```python
from build123d import *

# Parameters (mm, degrees)
F1_DEPTH = 25


with BuildPart() as f1:
    # F0 (on Right) → F1 (new body, symmetric)
    with BuildSketch(Plane.YZ):
        Polygon((-25, 0), (25, 0), (25, 45), (44.870459, 45), (44.870459, 60), (25, 60), (17, 103.547319), (25, 103.547319), (25, 121.547319), (-5, 121.547319), (-25, 91.547319), align=None)
    extrude(amount=F1_DEPTH, both=True)


solid = f1.part
```
Geometry: final body of the model. Coordinates: model frame, mm. A direction names the side the tool comes from. Coordinates: 2 decimals unless noted, no trailing zeros. Write each loop counter-clockwise with the first axis right and the second up, starting at its lowest first coordinate (ties: lowest second). Pieces come first, ordered by that corner, then holes. Notation, with made-up numbers: M 3,31 L 24,31 A29 ccw 24,62 Z; hole C 5.5,-25 d10. An arc over 180 degrees is marked long. Answer as CSV lines item,"result". Start each with the question number.
Q1. Cut plane B-B on x = -20.5. Return the cut outline in (y, z), then the cut area to 3 significant figures.
Q2. Reachability of faces 4 (the flat face through (0, 25, 22)), 5 (the flat face through (0.35, 21.056, 81.469)), 6 (the flat face through (0, 25, 112)), 7 (the flat face through (25, 2, 62)), 8 (the flat face through (0, 0, 0)) from +Z, -Z, +X, -X, +Y, -Y: full face, straight path, thin tool, end or side. Return the list, or none.
Q3. Pin query (flat end, axial travel): P1, Ø1, axis at x = 10.5, z = 85.5, coming from the +Y side; P2, Ø5.5, axis at x = 11, z = 115, coming from the +Y side; P3, Ø10, axis at x = 9, y = 35.5, coming from the -Z side. Return the tip coordinate at first contact, or that it passes through.
Q4. Line query: line 1 (Y direction, x = -6, z = 9.5); line 2 (Z direction, x = -7, y = 37); line 3 (Z direction, x = 23, y = -16). Output: solid intervals per line, ascending. Write a range as from..to.
Q5. Cut plane D-D on y = -7.5. Return the cut outline in (x, z), then the cut area to 3 significant figures.
Q6. Cut plane A-A on y = 19. Return the cut outline in (x, z), then the cut area to 3 significant figures.
Q7. Mould query, pull axis Z, two halves, no side actions, for faces 1 (the flat face through (0, 21, 103.547)), 2 (the flat face through (0, 44.87, 52)), 3 (the flat face through (0, 10, 121.547)). Classes: released by +Z, released by -Z, zero draft, split by the parting line, or undercut.
Q8. Cut plane C-C on z = 22. Return the cut outline in (x, y).
Findings below:
1,outline,"M -25,0 L 25,0 L 25,45 L 44.87,45 L 44.87,60 L 25,60 L 17,103.55 L 25,103.55 L 25,121.55 L -5,121.55 L -25,91.55 Z"
1,area,"5,900 mm2"
2,face 4,"-Z, +X, -X, +Y"
2,face 5,"+X, -X, +Y"
2,face 6,"+Z, +X, -X, +Y"
2,face 7,"+Z, -Z, +X, +Y, -Y"
2,face 8,"-Z, +X, -X, +Y, -Y"
3,P1,"stops at y = 20.41"
3,P2,"stops at y = 25"
3,P3,"stops at z = 45"
4,line 1,"y = -25..25"
4,line 2,"z = 45..60"
4,line 3,"z = 0..105.05"
5,outline,"M -25,0 L 25,0 L 25,117.8 L -25,117.8 Z"
5,area,"5,890 mm2"
6,outline,"M -25,0 L 25,0 L 25,92.66 L -25,92.66 Z; M -25,103.55 L 25,103.55 L 25,121.55 L -25,121.55 Z"
6,area,"5,530 mm2"
7,face 1,"undercut"
7,face 2,"zero draft"
7,face 3,"released by +Z"
8,outline,"M -25,-25 L 25,-25 L 25,25 L -25,25 Z"
